Could you check a few things on this drawing? It's one solid part, dimensions in mm from its lowest x, y, z. Give positions to 0.01 mm unless a question says otherwise; leave off trailing zeros. Loops run counter-clockwise (first coordinate to the right, second up) from the corner with the lowest first, then second, coordinate; pieces in that order, holes last.
1. Imagine slicing it at B-B (z = 9.5). List the corners of the cut face in (x, y) for me, plus the area to 3 significant figures.
2. Thinking about a two-plate mould opening in Z: for the marked faces 1, 2 and 3, which applies, +Z half, -Z half, draft (parallel to the pull), parting line (faces both ways), or undercut?
3. Imagine slicing it at C-C (y = 0.4). List the corners of the cut face in (x, z) for me, plus the area to 3 significant figures.
4. Imagine slicing it at D-D (y = 3.2). List the corners of the cut face in (x, z) for me, plus the area to 3 significant figures.
5. Imagine slicing it at A-A (x = 9.5). List the corners of the cut face in (y, z) for me, plus the area to 3 significant figures.
6. I need wall thicknesses on line 1 along Y through (x, z) = (14.25, 16); line 2 along X through (y, z) = (2.55, 2); line 3 along Z through (x, y) = (7.5, 1.5). Which ranges of each line are inside material? Lowest first, please.
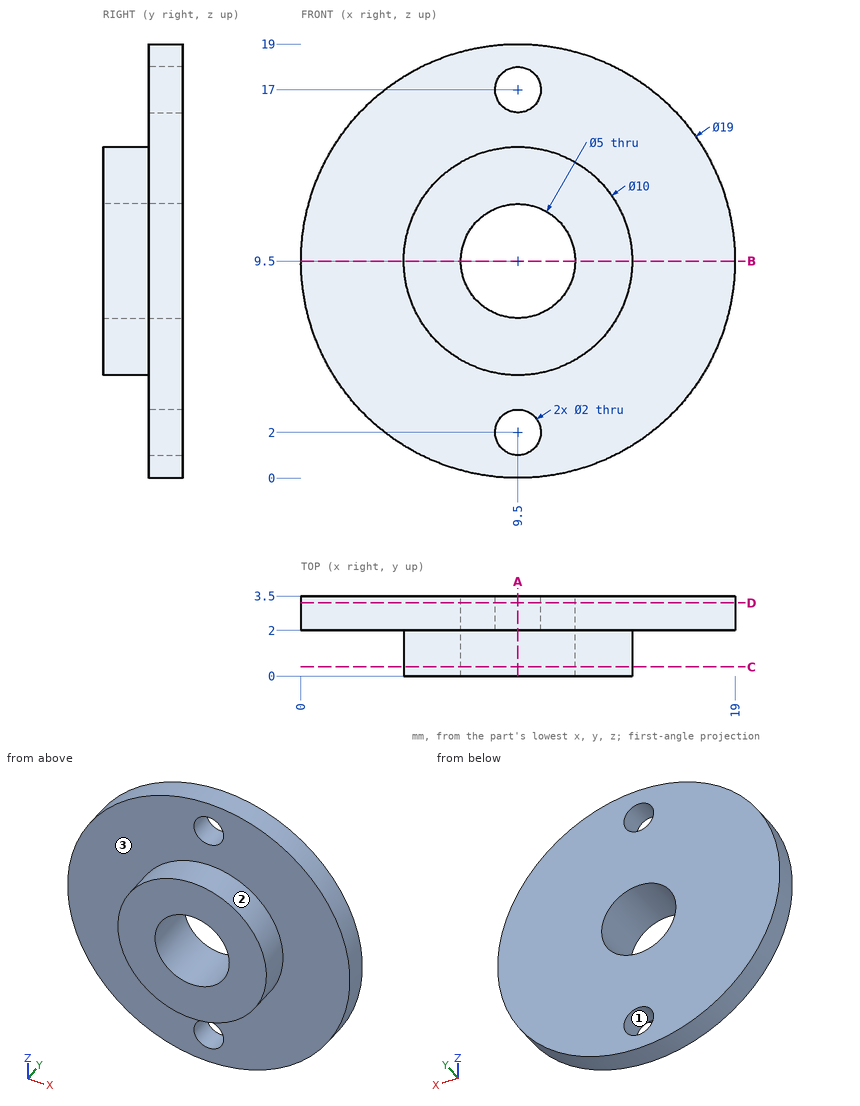
Derived:
1. outline: (0, 2) - (4.5, 2) - (4.5, 0) - (7, 0) - (7, 3.5) - (0, 3.5) - close; (12, 0) - (14.5, 0) - (14.5, 2) - (19, 2) - (19, 3.5) - (12, 3.5) - close
1. area: 31.0 mm2
2. face 1: undercut
2. face 2: parting line
2. face 3: draft
3. outline: circle Ø10 at (9.5, 9.5); hole circle Ø5 at (9.5, 9.5)
3. area: 58.9 mm2
4. outline: circle Ø19 at (9.5, 9.5); hole circle Ø5 at (9.5, 9.5); hole circle Ø2 at (9.5, 2); hole circle Ø2 at (9.5, 17)
4. area: 258 mm2
5. outline: (0, 4.5) - (2, 4.5) - (2, 3) - (3.5, 3) - (3.5, 7) - (0, 7) - close; (0, 12) - (3.5, 12) - (3.5, 16) - (2, 16) - (2, 14.5) - (0, 14.5) - close; (2, 0) - (3.5, 0) - (3.5, 1) - (2, 1) - close; (2, 18) - (3.5, 18) - (3.5, 19) - (2, 19) - close
5. area: 25.0 mm2
6. line 1: y = 2 to 3.5
6. line 2: x = 3.67 to 8.5, 10.5 to 15.33
6. line 3: z = 4.92 to 8, 11 to 14.08
